Geometry: final body of the model. Coordinates: model frame, mm. A direction names the side the tool comes from. Coordinates: 2 decimals unless noted, no trailing zeros. Order: outer loops, then holes, each group sorted by start corner. A loop starts at its lowest first (then second) coordinate and runs counter-clockwise, first axis right, second up. Notation, with made-up numbers: (55, -28) -> (104, -28) arc R28 cw to (104, -2) -> close; hole circle Ø11 at (80.5, 56). An arc over 180 degrees is marked (long way). Use one line per item in the form item = value.
```python
from build123d import *

# Parameters (mm, degrees)
SKETCH_1_R          = 4.75
EXTRUDE_1_DEPTH     = 6.5
SKETCH_2_R          = 6.5
EXTRUDE_2_DEPTH     = 1
EXTRUDE_START       = 1
SKETCH_3_R          = 6.5
EXTRUDE_3_DEPTH     = 1
SKETCH_4_R          = 1.75
CUT_EXTRUDE_1_DEPTH = 21


with BuildPart() as part:
    # 草图1 → 凸台-拉伸1 (new body)
    with BuildSketch(Plane.XY):
        with Locations(Location((0, 0, 0), (0, 0, 180))):
            Circle(SKETCH_1_R)
    extrude(amount=EXTRUDE_1_DEPTH)

    # 草图2 → 凸台-拉伸2 (add)
    with BuildSketch(Plane.XY.offset(6.5)):
        Circle(SKETCH_2_R)
    extrude(amount=EXTRUDE_2_DEPTH)

    # 草图3 → 凸台-拉伸3 (add)
    with BuildSketch(Plane(origin=(0, 0, 0), x_dir=(-1, 0, 0), z_dir=(0, 0, -1)).offset(EXTRUDE_START)):
        with Locations(Location((0, 0, 0), (0, 0, 180))):
            Circle(SKETCH_3_R)
    extrude(amount=-EXTRUDE_3_DEPTH)

    # 草图4 → 切除-拉伸1 (cut)
    with BuildSketch(Plane.XY.offset(7.5)):
        Circle(SKETCH_4_R)
    extrude(amount=-CUT_EXTRUDE_1_DEPTH, mode=Mode.SUBTRACT)


solid = part.part
```
1) Section D-D, the plane x = -0.75. Output: boundary loops of the cut face in (y, z).
Results found:
outline = (-6.46, -1) -> (-1.58, -1) -> (-1.58, 7.5) -> (-6.46, 7.5) -> (-6.46, 6.5) -> (-4.69, 6.5) -> (-4.69, 0) -> (-6.46, 0) -> close; (1.58, -1) -> (6.46, -1) -> (6.46, 0) -> (4.69, 0) -> (4.69, 6.5) -> (6.46, 6.5) -> (6.46, 7.5) -> (1.58, 7.5) -> close
2) Access query for faces 1 (the cylindrical face through (1.617, -0.67, 3.31)), 2 (the flat face through (0, -5, 6.5)). Directions: +Z, -Z, +X, -X, +Y, -Y. A direction counts if a zero-diameter tool reaches every point of the face in a straight line with its end or side. Return the directions, or none.
Results found:
face_1 = +Z, -Z
face_2 = none
3) Pull-direction query (Z, two-part tool) for faces 3 (the cylindrical face through (1.03, 4.637, 3.204)), 4 (the cylindrical face through (-5.158, -3.955, 6.993)), 5 (the flat face through (1.4, 1.4, -1)), 6 (the flat face through (0, 5, 0)); classes: released by +Z, released by -Z, zero draft, split by the parting line, or undercut.
Results found:
face_3 = undercut
face_4 = zero draft
face_5 = released by -Z
face_6 = undercut
4) Section B-B, the plane x = 5.5. Output: boundary loops of the cut face in (y, z).
Results found:
outline = (-3.46, -1) -> (3.46, -1) -> (3.46, 0) -> (-3.46, 0) -> close; (-3.46, 6.5) -> (3.46, 6.5) -> (3.46, 7.5) -> (-3.46, 7.5) -> close
5) Section A-A, the plane y = 0. Output: boundary loops of the cut face in (x, z), and give its area (3 significant figures).
Results found:
outline = (-6.5, -1) -> (-1.75, -1) -> (-1.75, 7.5) -> (-6.5, 7.5) -> (-6.5, 6.5) -> (-4.75, 6.5) -> (-4.75, 0) -> (-6.5, 0) -> close; (1.75, -1) -> (6.5, -1) -> (6.5, 0) -> (4.75, 0) -> (4.75, 6.5) -> (6.5, 6.5) -> (6.5, 7.5) -> (1.75, 7.5) -> close
area = 58.0 mm2
6) Contact query for flat-ended pins moving along their axis: P1, Ø3, axis at x = 0, y = 0, coming from the +Z side; P2, Ø1, axis at x = -1, z = 6.5, coming from the -Y side; P3, Ø5, axis at x = -4.5, z = 3.5, coming from the -Y side. Output: stop coordinate, or through.
Results found:
P1 = through
P2 = -6.48
P3 = -4.31
7) Material intervals for probe 1 along Y at (x, z) = (0, 4.5); probe 2 along Z at (x, y) = (-3, 5.25); probe 3 along X at (y, z) = (1, 6.75), sorted ascending. Write a range as from..to.
Results found:
probe_1 = -4.75..-1.75, 1.75..4.75
probe_2 = -1..0, 6.5..7.5
probe_3 = -6.42..-1.44, 1.44..6.42
8) Section C-C, the plane z = 2.75. Output: boundary loops of the cut face in (x, y), and give its area (3 significant figures).
Results found:
outline = circle Ø9.5 at (0, 0); hole circle Ø3.5 at (0, 0)
area = 61.3 mm2
